Here's how the part is built. I have some questions about the finished solid (model axes, mm). Face numbers are marked on the shaded views. A direction names the side the tool comes from. Coordinates: 2 decimals unless noted, no trailing zeros. Order: outer loops, then holes, each group sorted by start corner. A loop starts at its lowest first (then second) coordinate and runs counter-clockwise, first axis right, second up. Notation, with made-up numbers: (11.5, 19.25) -> (20.5, 19.25) arc R31 cw to (20.5, 45.25) -> close; hole circle Ø6 at (74.5, 59). An arc over 180 degrees is marked (long way). One line per item, written item: value. Start each with the question number.
```python
from build123d import *

# Parameters (mm, degrees)
CROQUIS1_R              = 30.5
SALIENTE_EXTRUIR1_DEPTH = 4
CORTAR_EXTRUIR3_START   = -4
CORTAR_EXTRUIR3_DEPTH   = 4
CORTAR_EXTRUIR6_START   = -10
CROQUIS9_R              = 2
CORTAR_EXTRUIR6_DEPTH   = 10
REDONDEO1_R             = 3
CROQUIS10_R             = 2
CORTAR_EXTRUIR7_DEPTH   = 4


with BuildPart() as part:
    # Croquis1 → Saliente-Extruir1 (new body)
    with BuildSketch(Plane(origin=(0, 0, 0), x_dir=(1, 0, 0), z_dir=(0, 1, 0))):
        with Locations(Location((0, 0, 0), (0, 0, 270))):
            Circle(CROQUIS1_R)
    extrude(amount=SALIENTE_EXTRUIR1_DEPTH)

    # Croquis5 → Cortar-Extruir3 (cut)
    with BuildSketch(Plane(origin=(0, 4, 0), x_dir=(1, 0, 0), z_dir=(0, 1, 0)).offset(CORTAR_EXTRUIR3_START)):
        with BuildLine():
            Line((28.814059068, 5), (30.087372767, 5))
            ThreePointArc((30.087372767, 5), (29.556634924, 7.526973624), (28.814059068, 10))
            Line((28.814059068, 10), (24.814059068, 10))
            Line((24.814059068, 10), (24.814059068, 5))
            Line((24.814059068, 5), (28.814059068, 5))
        make_face()
        with BuildLine():
            Line((30.087372767, -5), (28.814059068, -5))
            Line((28.814059068, -5), (24.814059068, -5))
            Line((24.814059068, -5), (24.814059068, -10))
            Line((24.814059068, -10), (28.814059068, -10))
            ThreePointArc((28.814059068, -10), (29.556634924, -7.526973624), (30.087372767, -5))
        make_face()
        with BuildLine():
            Line((-24.814059068, 5), (-24.814059068, 10))
            Line((-24.814059068, 10), (-28.814059068, 10))
            ThreePointArc((-28.814059068, 10), (-29.556634924, 7.526973624), (-30.087372767, 5))
            Line((-30.087372767, 5), (-28.814059068, 5))
            Line((-28.814059068, 5), (-24.814059068, 5))
        make_face()
        with BuildLine():
            Line((-28.814059068, -10), (-24.814059068, -10))
            Line((-24.814059068, -10), (-24.814059068, -5))
            Line((-24.814059068, -5), (-28.814059068, -5))
            Line((-28.814059068, -5), (-30.087372767, -5))
            ThreePointArc((-30.087372767, -5), (-29.556634924, -7.526973624), (-28.814059068, -10))
        make_face()
    extrude(amount=CORTAR_EXTRUIR3_DEPTH, mode=Mode.SUBTRACT)

    # Croquis9 → Cortar-Extruir6 (cut)
    with BuildSketch(Plane(origin=(0, 4, 0), x_dir=(1, 0, 0), z_dir=(0, 1, 0)).offset(CORTAR_EXTRUIR6_START)):
        Polygon((5.673284852, 12.685390231), (7.280253876, 10.770279124), (8.887222901, 8.855168016), (11.951400673, 11.426318455), (8.737462625, 15.25654067), align=None)
        Polygon((-10.796670675, -1.134543377), (-7.582732627, -4.964765592), (-4.518554854, -2.393615154), (-7.732492903, 1.436607062), align=None)
        with BuildLine():
            add(Edge.make_bspline(
                [(-10.646910399, -7.535916031), (-16.512406299, -9.080989315), (-22.046756553, -9.526586799), (-24.814059068, -5)],
                knots=[0.7678792, 0.7678792, 0.7678792, 0.7678792, 1, 1, 1, 1], degree=3))
            Line((-24.814059068, -5), (-24.814059068, -10))
            Line((-24.814059068, -10), (-28.814059068, -10))
            ThreePointArc((-28.814059068, -10), (-6.288730728, -29.84462876), (22.328940845, -20.776631121))
            add(Edge.make_bspline(
                [(22.328940845, -20.776631121), (5.973751648, -31.851207958), (18.415722084, 4.766196666), (-2.50799159, -5.391983749), (-10.646910399, -7.535916031)],
                knots=[0, 0, 0, 0, 0.445790092, 0.7678792, 0.7678792, 0.7678792, 0.7678792], degree=3))
        make_face()
        with BuildLine():
            add(Edge.make_bspline(
                [(-18.745320889, 15.664553597), (3.867000935, -2.576496257), (8.094246487, 2.496379136), (-8.307345659, 29.346856869)],
                knots=[0.040527546, 0.040527546, 0.040527546, 0.040527546, 1, 1, 1, 1], degree=3))
            ThreePointArc((-8.307345659, 29.346856869), (-20.930238649, 22.185019948), (-28.814059068, 10))
            Line((-28.814059068, 10), (-24.814059068, 10))
            add(Edge.make_bspline(
                [(-24.814059068, 10), (-24.456478323, 11.504954743), (-23.99064654, 12.985671633), (-23.418905183, 14.432273611)],
                knots=[0.635079884, 0.635079884, 0.635079884, 0.635079884, 0.831813486, 0.831813486, 0.831813486, 0.831813486], degree=3))
            ThreePointArc((-23.418905183, 14.432273611), (-21.393777069, 16.230440533), (-18.745320889, 15.664553597))
        make_face()
        Polygon((21.527275636, -8.931176939), (17.69705342, -12.145114987), (20.268203859, -15.20929276), (24.098426074, -11.995354711), align=None)
        with Locations(Location((2.550631881, 22.629718435, 0), (0, 0, 270))):
            Circle(CROQUIS9_R)
        with Locations(Location((18.138231416, 4.05314069, 0), (0, 0, 270))):
            Circle(CROQUIS9_R)
        with Locations(Location((-16.983501418, 6.238634388, 0), (0, 0, 270))):
            Circle(CROQUIS9_R)
        with Locations(Location((17.204026086, -17.780443199, 0), (0, 0, 270))):
            Circle(CROQUIS9_R)
    extrude(amount=CORTAR_EXTRUIR6_DEPTH, mode=Mode.SUBTRACT)

    # Redondeo1
    redondeo1_edges = [part.edges().sort_by_distance(p)[0] for p in [
        (-8.307345659, 2, -29.346856869),
    ]]
    fillet(redondeo1_edges, radius=REDONDEO1_R)

    # Croquis10 → Cortar-Extruir7 (cut)
    with BuildSketch(Plane(origin=(0, 4, 0), x_dir=(1, 0, 0), z_dir=(0, 1, 0))):
        with Locations(Location((-26.814059068, 0, 0), (0, 0, 270))):
            Circle(CROQUIS10_R)
        with Locations(Location((26.814059068, 0, 0), (0, 0, 270))):
            Circle(CROQUIS10_R)
    extrude(amount=-CORTAR_EXTRUIR7_DEPTH, mode=Mode.SUBTRACT)


solid = part.part
```
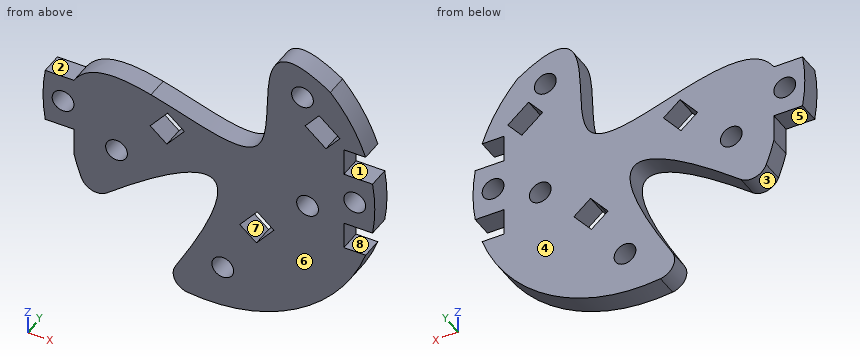
Q1. I need wall thicknesses on line 1 (X direction, y = 2.55, z = 0); line 2 (X direction, y = 0.3, z = 1.5); line 3 (X direction, y = 2.7, z = -10.5). Which ranges of each line are inside material? Lowest first, please.
Q2. Imagine slicing it at C-C (y = 1.55). Count the separate pieces of the cut face and the enclosed holes in it, plus the area to 3 significant figures.
Q3. Imagine slicing it at A-A (x = -26). Write out the boundary of the cut face in (y, z), plus the area to 3 significant figures.
Q4. Imagine slicing it at B-B (z = 0). Write out the boundary of the cut face in (x, y).
Q5. For the marked faces 4, 5, 6, 7 and 8, which set-ups out of +Z, -Z, +X, -X, +Y, -Y let a thin tool reach every point of the face, with its end or its side?
Q6. If we mould it in two halves opening along Z, with no side actions, what happens to the marked faces 1, 2 and 3? For each: +Z half, -Z half, draft (parallel to the pull), parting line (faces both ways), or undercut.
Q7. For P1, Ø1.2, axis at y = 2, z = -7.5, coming from the -X side; P2, Ø1.2, axis at x = 26, y = 1.5, coming from the +Z side; P3, Ø1.5, axis at x = -4, y = 3, coming from the +Z side; P4, Ø3.5, axis at x = 2.55, z = -22.63, coming from the +Y side, each with a flat end and sliding along its axis, tell me the tip position at first contact or that it passes through.
Completed:
1. line 1: x = -30.5 to -28.81, -24.81 to -9.44, -6.53 to 24.81, 28.81 to 30.5
1. line 2: x = -30.46 to -28.14, -25.49 to -10.49, -5.27 to 25.49, 28.14 to 30.46
1. line 3: x = -24.69 to -11.97, 1.12 to 7.51, 10.85 to 28.64
2. separate pieces: 1
2. enclosed holes: 9
2. area: 1,520 mm2
3. outline: (0, -5) -> (4, -5) -> (4, -1.83) -> (0, -1.83) -> close; (0, 1.83) -> (4, 1.83) -> (4, 5) -> (0, 5) -> close
3. area: 25.4 mm2
4. outline: (-30.5, 0) -> (-28.81, 0) -> (-28.81, 4) -> (-30.5, 4) -> close; (-24.81, 0) -> (-9.44, 0) -> (-9.44, 4) -> (-24.81, 4) -> close; (-6.53, 0) -> (24.81, 0) -> (24.81, 4) -> (-6.53, 4) -> close; (28.81, 0) -> (30.5, 0) -> (30.5, 4) -> (28.81, 4) -> close
5. face 4: +Z, -Z, +X, -X, +Y
5. face 5: -Z, -X, +Y, -Y
5. face 6: +Z, -Z, +X, -X, -Y
5. face 7: +Y, -Y
5. face 8: +X, +Y, -Y
6. face 1: undercut
6. face 2: +Z half
6. face 3: -Z half
7. P1: stops at x = -24.81
7. P2: stops at z = 16.88
7. P3: stops at z = 5.76
7. P4: passes through
